```python
from build123d import *

# Parameters (mm, degrees)
F0_R      = 44.45
F1_DEPTH  = 12.7
F3_DEPTH  = 12.7
F5_DEPTH  = 12.7
F7_DEPTH  = 25.4
F9_DEPTH  = 12.7
F10_R     = 3.175
F11_DEPTH = 12.7
F12_R     = 3.175


with BuildPart() as f1:
    # F0 (on Top) → F1 (new body)
    with BuildSketch(Plane.XY):
        Circle(F0_R)
    extrude(amount=F1_DEPTH)

    # F2 (on face) → F3 (cut)
    with BuildSketch(Plane.XY.offset(12.7)):
        with BuildLine():
            ThreePointArc((-28.575, -10.3124), (-18.2626, 0), (-28.575, 10.3124))
            Line((-28.575, 10.3124), (-43.2372166801, 10.3124))
            ThreePointArc((-43.2372166801, 10.3124), (-44.45, 0), (-43.2372166801, -10.3124))
            Line((-43.2372166801, -10.3124), (-28.575, -10.3124))
        make_face()
    extrude(amount=-F3_DEPTH, mode=Mode.SUBTRACT)

    # F4 (on face) → F5 (cut)
    with BuildSketch(Plane.XY.offset(12.7)):
        with BuildLine():
            Line((42.8275014446, 11.8999), (28.5877, 11.8999))
            ThreePointArc((28.5877, 11.8999), (16.6878, 0), (28.5877, -11.8999))
            Line((28.5877, -11.8999), (42.8275014446, -11.8999))
            ThreePointArc((42.8275014446, -11.8999), (44.45, 0), (42.8275014446, 11.8999))
        make_face()
    extrude(amount=-F5_DEPTH, mode=Mode.SUBTRACT)

    # F6 (on face) → F7 (cut)
    with BuildSketch(Plane.XY.offset(12.7)):
        with BuildLine():
            Line((-8.7249, 43.585302798), (-8.7249, 28.5877))
            ThreePointArc((-8.7249, 28.5877), (0, 19.8628), (8.7249, 28.5877))
            Line((8.7249, 28.5877), (8.7249, 43.585302798))
            ThreePointArc((8.7249, 43.585302798), (0, 44.45), (-8.7249, 43.585302798))
        make_face()
    extrude(amount=-F7_DEPTH, mode=Mode.SUBTRACT)

    # F8 (on face) → F9 (cut)
    with BuildSketch(Plane.XY.offset(12.7)):
        with BuildLine():
            ThreePointArc((7.1374, -28.575), (0, -21.4376), (-7.1374, -28.575))
            Line((-7.1374, -28.575), (-7.1374, -43.8732267019))
            ThreePointArc((-7.1374, -43.8732267019), (0, -44.45), (7.1374, -43.8732267019))
            Line((7.1374, -43.8732267019), (7.1374, -28.575))
        make_face()
    extrude(amount=-F9_DEPTH, mode=Mode.SUBTRACT)

    # F10 (on face) → F11 (cut, through all)
    with BuildSketch(Plane.XY.offset(12.7)):
        Circle(F10_R)
    extrude(amount=-F11_DEPTH, mode=Mode.SUBTRACT)

    # F12
    f12_edges = [f1.edges().sort_by_distance(p)[0] for p in [
        (42.827501, -11.8999, 6.35),
        (42.827501, 11.8999, 6.35),
        (8.7249, 43.585303, 6.35),
        (-8.7249, 43.585303, 6.35),
        (7.1374, -43.873227, 6.35),
        (-7.1374, -43.873227, 6.35),
        (-43.237217, -10.3124, 6.35),
        (-43.237217, 10.3124, 6.35),
    ]]
    fillet(f12_edges, radius=F12_R)


solid = f1.part
```
Geometry: final body of the model. Coordinates: model frame, mm. A direction names the side the tool comes from. Round coordinates to 2 decimals unless told otherwise and drop trailing zeros. Loops run counter-clockwise (first coordinate to the right, second up) from the corner with the lowest first, then second, coordinate; pieces in that order, holes last. Notation, with made-up numbers: (-13.5, -14) -> (34.5, -14) arc R29 ccw to (34.5, 24) -> close; hole circle Ø10 at (68.25, 35.25). An arc over 180 degrees is marked (long way). Write each question's results on one line, items separated by ' | '.
Item 1: Cut plane D-D on x = 15.5. Return the cut outline in (y, z), and give its area (3 significant figures).
Answers below:
outline: (-41.66, 0) -> (41.66, 0) -> (41.66, 12.7) -> (-41.66, 12.7) -> close | area: 1,060 mm²
Item 2: Pull-direction query (X, two-part tool) for faces 1 (the face through (33, -11.9, 6)), 2 (the face through (16.69, 0.26, 6.44)), 3 (the face through (-10.039, 42.095, 6.261)); classes: pulls with the +X half, pulls with the -X half, needs draft (parallel to the pull), parting line crosses it, or undercut.
Answers below:
face 1: needs draft | face 2: pulls with the +X half | face 3: undercut
Item 3: Cut plane A-A on y = 0. Return the cut outline in (x, z) (3 decimals).
Answers below:
outline: (-18.263, 0) -> (-3.175, 0) -> (-3.175, 12.7) -> (-18.263, 12.7) -> close; (3.175, 0) -> (16.688, 0) -> (16.688, 12.7) -> (3.175, 12.7) -> close
Item 4: Set-up query: faces 4 (the face through (-34, -10.312, 6)), 5 (the face through (34, 11.9, 6)), 6 (the face through (-7.137, -34, 6)). Return all of +Z, -Z, +X, -X, +Y, -Y with unobstructed straight access to the full face (end or side cutting, diameter ignored); none if empty.
Answers below:
face 4: +Z, -Z, -X | face 5: +Z, -Z, +X | face 6: +Z, -Z, -Y
Item 5: Cut plane C-C on x = 0. Return the cut outline in (y, z) (3 decimals).
Answers below:
outline: (-21.438, 0) -> (-3.175, 0) -> (-3.175, 12.7) -> (-21.438, 12.7) -> close; (3.175, 0) -> (19.863, 0) -> (19.863, 12.7) -> (3.175, 12.7) -> close
Item 6: Pin query (flat end, axial travel): pin 1 Ø3 at (x, z) = (-34, 7.5) entering from +Y; pin 2 Ø5.5 at (y, z) = (32.5, 6.5) entering from +X; pin 3 Ø1.5 at (x, z) = (30, 4) entering from -Y. Return the tip coordinate at first contact, or that it passes through.
Answers below:
pin 1: stops at y = 30.32 | pin 2: stops at x = 33.03 | pin 3: stops at y = -33.47
Item 7: Line query: probe 1 along Y at (x, z) = (0, 9.5) (3 decimals); probe 2 along Y at (x, z) = (26, 8.5); probe 3 along X at (y, z) = (-33, 10). Output: solid intervals per line, ascending. Write a range as [from, to].
Answers below:
probe 1: y = [-21.438, -3.175], [3.175, 19.863] | probe 2: y = [-36.05, -11.62], [11.62, 36.05] | probe 3: x = [-29.78, -7.14], [7.14, 29.78]
